Design review of the part shown in the three views and the two pictorial views. Dimensions are in mm from the part's minimum x, y and z. A direction names the side the tool comes from. Give positions to 0.01 mm unless a question says otherwise; leave off trailing zeros. Order: outer loops, then holes, each group sorted by start corner. A loop starts at its lowest first (then second) coordinate and runs counter-clockwise, first axis right, second up. Notation, with made-up numbers: (-16, -11) - (43, -11) arc R24 ccw to (43, 24) - close; hole circle Ø8 at (65.25, 57.5). An arc over 180 degrees is marked (long way). Put each result on its own line as item: value. Start each with the question number.
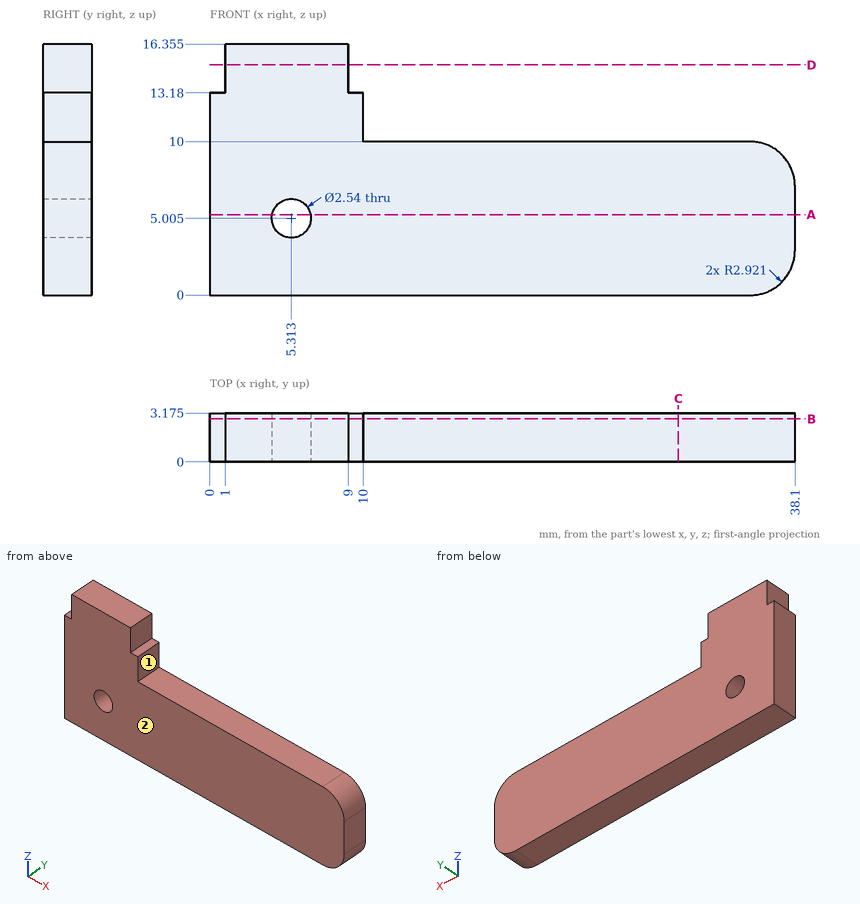
1. Add section D-D, the plane z = 15. Give the boundary of the cut face in (x, y) (3 decimals).
2. Add section B-B, the plane y = 2.8. Give the boundary of the cut face in (x, z) (3 decimals), then the cut area to 3 significant figures.
3. Wall thickness on line 1 (X direction, y = 0.9, z = 10.25); line 2 (X direction, y = 2.35, z = 4): over which ranges is each line inside the solid? List them lowest first. Write a range as from..to.
4. Add section C-C, the plane x = 30.5. Give the boundary of the cut face in (y, z) (3 decimals), then the cut area to 4 significant figures.
5. Clearance check with flat-ended pins moving along their axes: pin 1 (0.5 mm diameter, centred on x = 0.5, y = 2.5, fed in from +Z); pin 2 (1 mm diameter, centred on y = 1, z = 12, fed in from +X). State where each tip first meets the part, or that it passes through.
6. Tool access review of the marked faces 1 and 2: name each direction out of +Z, -Z, +X, -X, +Y, -Y from which nothing blocks a thin tool from reaching the whole face with its end or side.
7. Add section A-A, the plane z = 5.25. Give the boundary of the cut face in (x, y) (3 decimals), then the cut area to 3 significant figures.
Found:
1. outline: (1, 0) - (9, 0) - (9, 3.175) - (1, 3.175) - close
2. outline: (0, 0) - (35.179, 0) arc R2.921 ccw to (38.1, 2.921) - (38.1, 7.079) arc R2.921 ccw to (35.179, 10) - (10, 10) - (10, 13.18) - (9, 13.18) - (9, 16.355) - (1, 16.355) - (1, 13.18) - (0, 13.18) - close; hole circle Ø2.54 at (5.313, 5.005)
2. area: 429 mm^2
3. line 1: x = 0..10
3. line 2: x = 0..4.54, 6.09..38.1
4. outline: (0, 0) - (3.175, 0) - (3.175, 10) - (0, 10) - close
4. area: 31.75 mm^2
5. pin 1: stops at z = 13.18
5. pin 2: stops at x = 10
6. face 1: +Z, +X, +Y, -Y
6. face 2: +Z, -Z, +X, -X, -Y
7. outline: (0, 0) - (4.067, 0) - (4.067, 3.175) - (0, 3.175) - close; (6.559, 0) - (38.1, 0) - (38.1, 3.175) - (6.559, 3.175) - close
7. area: 113 mm^2
